Check sheet for the drawn part. Datum: minimum x, y, z corner. Units: mm. A direction names the side the tool comes from. Coordinates: 2 decimals unless noted, no trailing zeros. Loops run counter-clockwise (first coordinate to the right, second up) from the corner with the lowest first, then second, coordinate; pieces in that order, holes last. Notation, with made-up numbers: (17.25, -17) - (53.25, -17) arc R24 ccw to (53.25, 15) - close; hole circle Ø7 at (66, -26.75). An arc over 180 degrees is marked (long way). Answer as CSV lines item,"result". Start each with the question number.
1. Cross-section at D-D (z = 54). Enter the section's corners in (x, y), plus the area to 3 significant figures.
2. Set-up check for the marked faces 1, 2, 3 and 4: record each of +Z, -Z, +X, -X, +Y, -Y from which the full face is reachable in a straight line by a thin tool's end or side.
3. Cross-section at C-C (y = 40.5). Enter the section's corners in (x, z), plus the area to 3 significant figures.
4. Material ranges on line 1 (X direction, y = 71, z = 51); line 2 (Y direction, x = 45, z = 22); line 3 (X direction, y = 5, z = 42), recorded low to high. Write a range as [from, to].
5. Release check for a two-part mould opening along X. For the marked faces 5, 6, 7 and 8 record: pulls with the +X half, pulls with the -X half, needs draft (parallel to the pull), parting line crosses it, or undercut.
6. Cross-section at B-B (z = 23). Enter the section's corners in (x, y).
7. Cross-section at A-A (y = 58). Enter the section's corners in (x, z).
8. Gauge pin test, flat end, axial feed: P1, Ø12.5, axis at x = 7, z = 61, coming from the -Y side. Record the tip position at first contact, or that the pin passes through.
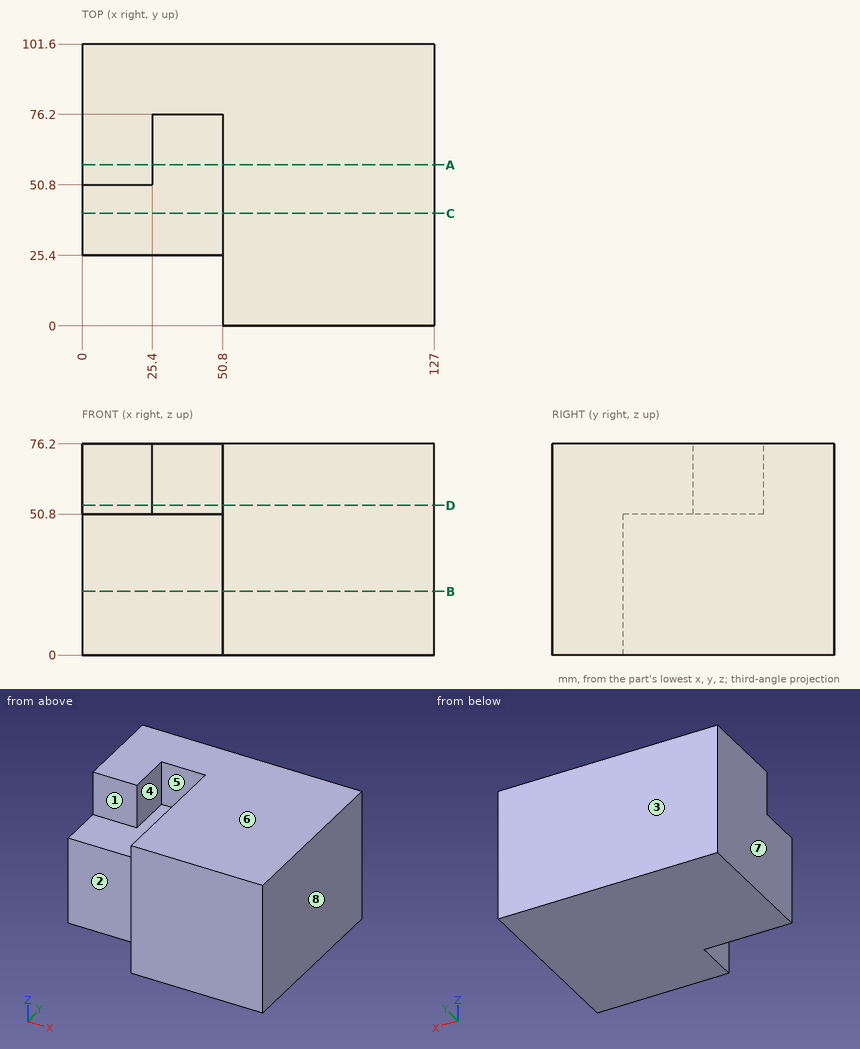
Values follow:
1,outline,"(0, 50.8) - (25.4, 50.8) - (25.4, 76.2) - (50.8, 76.2) - (50.8, 0) - (127, 0) - (127, 101.6) - (0, 101.6) - close"
1,area,"9,680 mm²"
2,face 1,"+Z, -X, -Y"
2,face 2,"+Z, -Z, -X, -Y"
2,face 3,"+Z, -Z, +X, -X, +Y"
2,face 4,"+Z, -Y"
3,outline,"(0, 0) - (127, 0) - (127, 76.2) - (50.8, 76.2) - (50.8, 50.8) - (0, 50.8) - close"
3,area,"8,390 mm²"
4,line 1,"x = [0, 25.4], [50.8, 127]"
4,line 2,"y = [25.4, 101.6]"
4,line 3,"x = [50.8, 127]"
5,face 5,"undercut"
5,face 6,"needs draft"
5,face 7,"pulls with the -X half"
5,face 8,"pulls with the +X half"
6,outline,"(0, 25.4) - (50.8, 25.4) - (50.8, 0) - (127, 0) - (127, 101.6) - (0, 101.6) - close"
7,outline,"(0, 0) - (127, 0) - (127, 76.2) - (50.8, 76.2) - (50.8, 50.8) - (25.4, 50.8) - (25.4, 76.2) - (0, 76.2) - close"
8,P1,"stops at y = 50.8"
